CAD build for the part. Positions are in the model's coordinates, mm. Face numbers are marked on the shaded views. A direction names the side the tool comes from. Round coordinates to 2 decimals unless told otherwise and drop trailing zeros. Loops run counter-clockwise (first coordinate to the right, second up) from the corner with the lowest first, then second, coordinate; pieces in that order, holes last. Notation, with made-up numbers: M 64.25,72.5 L 93.25,72.5 A23 cw 93.25,86.5 Z; hole C 84,80 d9. An arc over 180 degrees is marked long. Use a Markdown table: item, result. Add a question column.
(1) Flat gauge pins, fed straight in: P1, Ø10, axis at x = -5, z = -6.5, coming from the +Y side; P2, Ø4.5, axis at x = -64.5, y = -6, coming from the -Z side; P3, Ø8, axis at y = 3, z = -21, coming from the -X side. Where does each tip first touch, or does it go through?
(2) Wall check: L1, parallel to Y at x = -8, z = -10; L2, parallel to X at y = -5, z = 0; L3, parallel to X at y = -11.75, z = -4. Give the ranges that are in metal, low to high.
(3) Two-plate mould, pull along X, no slides. Class the marked faces 1, 2 and 3: released by +X, released by -X, zero draft, split by the parting line, or undercut.
(4) Which spindle directions (+Z, -Z, +X, -X, +Y, -Y) get a long thin tool onto all of the face, cutting with end or side? Do the marked faces 4, 5, 6 and 7. Say none if no direction does.
(5) Band-saw the part on C-C, the plane y = 6. Write the cut outline in (x, z).
(6) Band-saw the part on D-D, the plane z = -18. Write the cut outline in (x, y), and give its area (3 significant figures).
(7) Band-saw the part on A-A, the plane z = 12. Write the cut outline in (x, y), and give its area (3 significant figures).
(8) Band-saw the part on B-B, the plane x = -38.5. Write the cut outline in (y, z), and give its area (3 significant figures).
from build123d import *

# Parameters (mm, degrees)
F1_DEPTH = 9
F4_R     = 5
F5_R     = 5


with BuildPart() as f1:
    # F0 (on Front) → F1 (new body)
    with BuildSketch(Plane.XZ):
        with BuildLine():
            Line((35, -30), (35, 30))
            Line((35, 30), (-7.4289321881, 30))
            Line((-7.4289321881, 30), (-30, 7.4289321881))
            ThreePointArc((-30, 7.4289321881), (-33.2442334882, 5.2612046749), (-37.0710678119, 4.5))
            Line((-37.0710678119, 4.5), (-62.9289321881, 4.5))
            Line((-62.9289321881, 4.5), (-62.9289321881, -4.5))
            Line((-62.9289321881, -4.5), (-37.0710678119, -4.5))
            ThreePointArc((-37.0710678119, -4.5), (-33.2442334882, -5.2612046749), (-30, -7.4289321881))
            Line((-30, -7.4289321881), (-7.4289321881, -30))
            Line((-7.4289321881, -30), (35, -30))
        make_face()
    extrude(amount=F1_DEPTH)

    # F2 (on face) → F3 (revolve)
    with BuildSketch(Plane(origin=(-62.9289321881, 0, 0), x_dir=(0, -1, 0), z_dir=(-1, 0, 0))):
        with BuildLine():
            Line((3.679, -4.5), (3.679, -14.142))
            ThreePointArc((3.679, -14.142), (17.821, 0), (3.679, 14.142))
            Line((3.679, 14.142), (3.679, 4.5))
            Line((3.679, 4.5), (9, 4.5))
            Line((9, 4.5), (9, -4.5))
            Line((9, -4.5), (3.679, -4.5))
        make_face()
    revolve(axis=Axis((-62.9289321881, -3.679, 0), (0, 0, -1)))

    # F4
    f4_edges = [f1.edges().sort_by_distance(p)[0] for p in [
        (-49.550362, -4.550796, 4.5),
        (-49.273855, 0, 0),
        (-49.550362, -4.550796, -4.5),
        (-49.826142, -9, 0),
    ]]
    fillet(f4_edges, radius=F4_R)

    # F5
    f5_edges = [f1.edges().sort_by_distance(p)[0] for p in [
        (35, -4.5, -30),
        (35, -4.5, 30),
        (-7.428932, -4.5, 30),
        (-7.428932, -4.5, -30),
    ]]
    fillet(f5_edges, radius=F5_R)


solid = f1.part
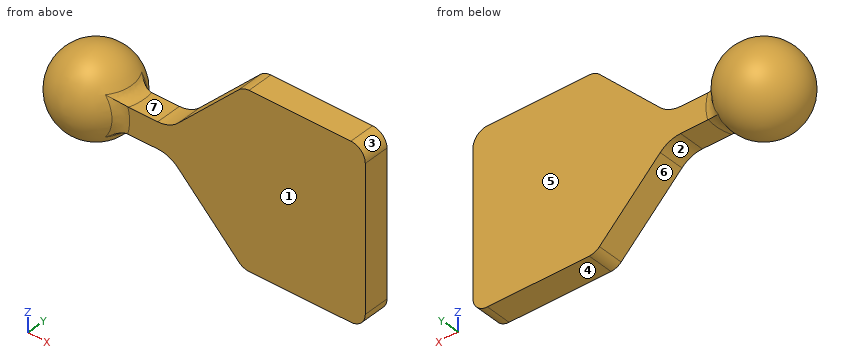
Return value:
| question | item | result |
|---|---|---|
| 1 | P1 | y = 0 |
| 1 | P2 | z = -14.13 |
| 1 | P3 | x = -19.07 |
| 2 | L1 | -9 to 0 |
| 2 | L2 | -77.01 to -68.08, -62.93 to 35 |
| 2 | L3 | -73.83 to -52.03 |
| 3 | face 1 | zero draft |
| 3 | face 2 | undercut |
| 3 | face 3 | released by +X |
| 4 | face 4 | -Z, +X, -X, +Y, -Y |
| 4 | face 5 | +Z, -Z, +X, +Y |
| 4 | face 6 | -Z, +Y, -Y |
| 4 | face 7 | +Z, +Y, -Y |
| 5 | outline | C -62.93,0 d20.62 |
| 6 | outline | M -19.43,-9 L 35,-9 L 35,0 L -19.43,0 Z |
| 6 | area | 490 mm^2 |
| 7 | outline | C -62.93,-3.68 d14.97; M -25.43,-9 L 35,-9 L 35,0 L -25.43,0 Z |
| 7 | area | 720 mm^2 |
| 8 | outline | M -9,-4.5 L 0,-4.5 L 0,4.5 L -9,4.5 Z |
| 8 | area | 81.0 mm^2 |
